```python
from build123d import *

# Parameters (mm, degrees)
F0_R     = 58.1684180137
F0_R_2   = 44.7813841063
F1_DEPTH = 25.4
F2_SIZE  = 10.16


# Not quite as in the source:
# - a fillet or chamfer that OpenCascade refuses, or shapes differently, is made with other operations: its cross-section is extruded or revolved along the edge and cut away or added


with BuildPart() as f1:
    # F0 (on Front) → F1 (new body)
    with BuildSketch(Plane.XZ):
        Circle(F0_R)
        Circle(F0_R_2, mode=Mode.SUBTRACT)
    extrude(amount=F1_DEPTH)

    # F2
    f2_edges = [f1.edges().sort_by_distance(p)[0] for p in [
        (-44.781384, -25.4, 0),
    ]]
    chamfer(f2_edges, length=F2_SIZE)

    # F3: fillet of radius 5.08 on 2 edges, made by hand

    # F3_s1 → F3_t2 (revolve, cut)
    with BuildSketch(Plane.XY):
        with BuildLine():
            ThreePointArc((54.9413841063, -25.4), (57.2848133567, -23.5329802725), (58.1684180137, -20.669998239))
            Line((58.1684180137, -20.669998239), (58.1684180137, -25.4))
            Line((58.1684180137, -25.4), (54.9413841063, -25.4))
        make_face()
    revolve(axis=Axis((0, -25.4, 0), (0, -1, 0)), mode=Mode.SUBTRACT)

    # F3_s3 → F3_t4 (revolve, cut)
    with BuildSketch(Plane.XY):
        with BuildLine():
            ThreePointArc((53.0884180137, 0), (56.6805204621, -1.4878975516), (58.1684180137, -5.08))
            Line((58.1684180137, -5.08), (58.1684180137, 0))
            Line((58.1684180137, 0), (53.0884180137, 0))
        make_face()
    revolve(axis=Axis((0, 0, 0), (0, -1, 0)), mode=Mode.SUBTRACT)


solid = f1.part
```
Could you check a few things on this model? Use its own coordinates, in mm. Coordinates: 2 decimals unless noted, no trailing zeros. Order: outer loops, then holes, each group sorted by start corner. A loop starts at its lowest first (then second) coordinate and runs counter-clockwise, first axis right, second up. Notation, with made-up numbers: M -9,70.5 L 12,70.5 A10 cw 12,77.5 Z; hole C -6,-3 d1. An arc over 180 degrees is marked long. Use one line per item in the form item = value. Start each with the question number.
1. Suppose I cut it at C-C on y = -13.5. Write out the boundary of the cut face in (x, z), then the cut area to 3 significant figures.
2. Suppose I cut it at D-D on y = -2.5. Write out the boundary of the cut face in (x, z).
3. Suppose I cut it at A-A on x = 0. Write out the boundary of the cut face in (y, z), then the cut area to 3 significant figures.
4. Suppose I cut it at B-B on z = 0. Write out the boundary of the cut face in (x, y).
5. For pin 1 (6 mm diameter, centred on x = 25.5, y = -19, fed in from -Z); pin 2 (1 mm diameter, centred on x = 36, z = 40.5, fed in from -Y); pin 3 (2 mm diameter, centred on y = -7, z = 38, fed in from -X), each with a flat end and sliding along its axis, tell me the tip position at first contact or that it passes through.
6. We'd pull the mould along X, two halves only. Please class faces 1 (the flat face through (-24, 0, -39)), 2 (the cylindrical face through (-5.83, -7.51, 44.4)), 3 (the cylindrical face through (55.482, -12.766, 17.472)): +X half, -X half, draft (parallel to the pull), parting line (faces both ways), or undercut.
7. Please list where these lines run through material, in increasing order: line 1 (Z direction, x = 0, y = -5); line 2 (X direction, y = -11.5, z = 1); line 3 (X direction, y = -10, z = 5).
Geometry says:
q1.outline = C 0,0 d116.34; hole C 0,0 d89.56
q1.area = 4,330 mm^2
q2.outline = C 0,0 d114.93; hole C 0,0 d89.56
q3.outline = M -25.4,-54.94 A5.08 ccw -20.67,-58.17 L -5.08,-58.17 A5.08 ccw 0,-53.09 L 0,-44.78 L -15.24,-44.78 Z; M -25.4,54.94 L -15.24,44.78 L 0,44.78 L 0,53.09 A5.08 ccw -5.08,58.17 L -20.67,58.17 A5.08 ccw Z
q3.area = 557 mm^2
q4.outline = M -58.17,-20.67 A5.08 ccw -54.94,-25.4 L -44.78,-15.24 L -44.78,0 L -53.09,0 A5.08 ccw -58.17,-5.08 Z; M 44.78,-15.24 L 54.94,-25.4 A5.08 ccw 58.17,-20.67 L 58.17,-5.08 A5.08 ccw 53.09,0 L 44.78,0 Z
q5.pin_1 = -53.64
q5.pin_2 = -25.15
q5.pin_3 = -44.88
q6.face_1 = draft
q6.face_2 = undercut
q6.face_3 = parting line
q7.line_1 = -58.17 to -44.78, 44.78 to 58.17
q7.line_2 = -58.16 to -44.77, 44.77 to 58.16
q7.line_3 = -57.95 to -44.5, 44.5 to 57.95
